from build123d import *

# Parameters (mm, degrees)
F0_R      = 5
F1_DEPTH  = 2
F2_R      = 4
F3_DEPTH  = 8
F4_R      = 6
F5_DEPTH  = 2
F7_DEPTH  = 2.5
F10_DEPTH = 8
F11_SIZE  = 1
F8_R      = 4
F8_R_2    = 3
F12_DEPTH = 3.1
F13_R     = 5
F13_R_2   = 4
F13_R_3   = 3
F14_DEPTH = 2
F16_DEPTH = 6
F17_SIZE  = 0.99999


# Not quite as in the source:
# - a fillet or chamfer is up to 0.001 mm smaller than in the source, because OpenCascade refuses the exact size


with BuildPart() as f1:
    # F0 (on Top) → F1 (new body)
    with BuildSketch(Plane.XY):
        Circle(F0_R)
    extrude(amount=F1_DEPTH)

    # F2 (on face) → F3 (join)
    with BuildSketch(Plane.XY.offset(2)):
        Circle(F2_R)
    extrude(amount=F3_DEPTH)

    # F4 (on face) → F5 (join)
    with BuildSketch(Plane.XY.offset(10)):
        Circle(F4_R)
    extrude(amount=F5_DEPTH)

    # F6 (on face) → F7 (join)
    with BuildSketch(Plane.XY.offset(12)):
        with BuildLine():
            ThreePointArc((6, 0), (5.9789831367, 0.5017575617), (5.9160797831, 1))
            Line((5.9160797831, 1), (4.5160797831, 1))
            Line((4.5160797831, 1), (4.5160797831, -1))
            Line((4.5160797831, -1), (5.9160797831, -1))
            ThreePointArc((5.9160797831, -1), (5.9789831367, -0.5017575617), (6, 0))
        make_face()
        with BuildLine():
            Line((-4.5160797831, 1), (-5.9160797831, 1))
            ThreePointArc((-5.9160797831, 1), (-6, 0), (-5.9160797831, -1))
            Line((-5.9160797831, -1), (-4.5160797831, -1))
            Line((-4.5160797831, -1), (-4.5160797831, 1))
        make_face()
    extrude(amount=F7_DEPTH)

    # F9 (on face) → F10 (cut)
    with BuildSketch(Plane(origin=(0, 0, 0), x_dir=(1, 0, 0), z_dir=(0, 0, -1))):
        with BuildLine():
            ThreePointArc((1.6, 2.6), (0, 3.0528675045), (-1.6, 2.6))
            Line((-1.6, 2.6), (-1.6, -2.6))
            ThreePointArc((-1.6, -2.6), (0, -3.0528675045), (1.6, -2.6))
            Line((1.6, -2.6), (1.6, 2.6))
        make_face()
    extrude(amount=-F10_DEPTH, mode=Mode.SUBTRACT)

    # F11
    f11_edges = [f1.edges().sort_by_distance(p)[0] for p in [
        (-5, 0, 0),
    ]]
    chamfer(f11_edges, length=F11_SIZE)

    # F8 (on face) → F12 (join)
    with BuildSketch(Plane.XY.offset(12)):
        Circle(F8_R)
        Circle(F8_R_2, mode=Mode.SUBTRACT)
    extrude(amount=F12_DEPTH)

    # F13 (on face) → F14 (join)
    with BuildSketch(Plane.XY.offset(15.1)):
        Circle(F13_R)
        Circle(F13_R_2, mode=Mode.SUBTRACT)
        Circle(F13_R_2)
        Circle(F13_R_3, mode=Mode.SUBTRACT)
    extrude(amount=F14_DEPTH)

    # F15 (on face) → F16 (cut)
    with BuildSketch(Plane.XY.offset(17.1)):
        with BuildLine():
            Line((-2.8284271247, 1), (-4.8989794856, 1))
            ThreePointArc((-4.8989794856, 1), (-5, 0), (-4.8989794856, -1))
            Line((-4.8989794856, -1), (-2.8284271247, -1))
            ThreePointArc((-2.8284271247, -1), (-3, 0), (-2.8284271247, 1))
        make_face()
        with BuildLine():
            ThreePointArc((0.9908586892, 4.9008365672), (-0.0278443772, 4.9999224685), (-1.0453806817, 4.8894968279))
            Line((-1.0453806817, 4.8894968279), (-1.0261823806, 2.819033473))
            ThreePointArc((-1.0261823806, 2.819033473), (-0.0085441177, 2.999987833), (1.0101083624, 2.8248329324))
            Line((1.0101083624, 2.8248329324), (0.9908586892, 4.9008365672))
        make_face()
        with BuildLine():
            ThreePointArc((5, 0), (4.974680765, 0.50254481), (4.8989794856, 1))
            Line((4.8989794856, 1), (2.8284271247, 1))
            ThreePointArc((2.8284271247, 1), (2.956795679, 0.5073059362), (3, 0))
            ThreePointArc((3, 0), (2.956795679, -0.5073059362), (2.8284271247, -1))
            Line((2.8284271247, -1), (4.8989794856, -1))
            ThreePointArc((4.8989794856, -1), (4.974680765, -0.50254481), (5, 0))
        make_face()
        with BuildLine():
            Line((-0.9737316464, -2.8375776079), (-0.9545333452, -4.9080409628))
            ThreePointArc((-0.9545333452, -4.9080409628), (0.0648756616, -4.9995790971), (1.0815661863, -4.8816200779))
            Line((1.0815661863, -4.8816200779), (1.0623165131, -2.8056164431))
            ThreePointArc((1.0623165131, -2.8056164431), (0.0470871391, -2.9996304441), (-0.9737316464, -2.8375776079))
        make_face()
    extrude(amount=-F16_DEPTH, mode=Mode.SUBTRACT)

    # F17 (size 1 in the source; OpenCascade refuses exactly that, so slightly less here)
    f17_edges = [f1.edges().sort_by_distance(p)[0] for p in [
        (3.564895, -3.505927, 15.1),
        (-3.551887, 3.519105, 15.1),
        (-3.519105, -3.551887, 15.1),
        (3.564895, -3.505927, 17.1),
        (-3.519105, -3.551887, 17.1),
        (-3.551887, 3.519105, 17.1),
        (3.532234, 3.53883, 17.1),
        (3.532234, 3.53883, 15.1),
    ]]
    chamfer(f17_edges, length=F17_SIZE)


solid = f1.part
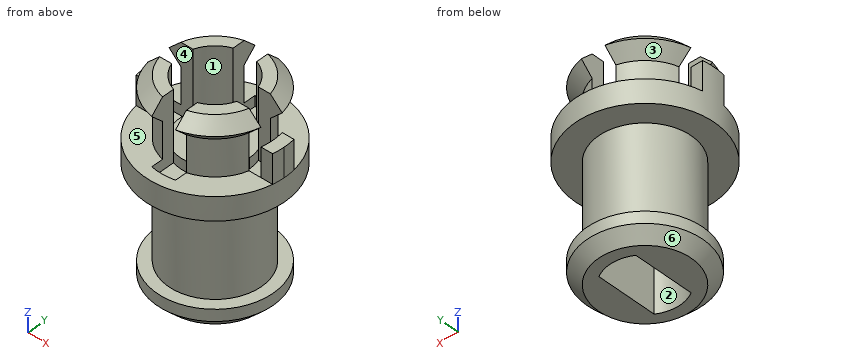
Can you work these out from the model? Positions are in its coordinate system, mm. Face numbers are marked on the shaded views. A direction names the side the tool comes from. Give positions to 0.01 mm unless a question says otherwise; leave off trailing zeros. Write each loop counter-clockwise with the first axis right and the second up, starting at its lowest first coordinate (ties: lowest second). Pieces come first, ordered by that corner, then holes. Notation, with made-up numbers: (-3, 57.5) -> (32, 57.5) arc R24 cw to (32, 70.5) -> close; hole circle Ø2 at (-4.75, 69). An arc over 180 degrees is marked (long way). Answer as a JSON object with one key per item and string values. Group by question number.
Item 1: We'd pull the mould along Z, two halves only. Please class the marked faces 4, 5 and 6: +Z half, -Z half, draft (parallel to the pull), parting line (faces both ways), or undercut.
Item 2: Please list where these lines run through material, in increasing order: line 1 (X direction, y = -4.25, z = 11.25); line 2 (Y direction, x = 2.5, z = 15.25); line 3 (Z direction, x = 5.25, y = -2.25). Write a range as [from, to].
Item 3: For the marked faces 1, 2 and 3, which set-ups out of +Z, -Z, +X, -X, +Y, -Y let a thin tool reach every point of the face, with its end or its side?
Item 4: Suppose I cut it at A-A (z = 2.25). Please give me the cut outline in (x, y).
Item 5: Suppose I cut it at C-C (z = 9.75). Please give me the cut outline in (x, y).
Item 6: Suppose I cut it at B-B (x = 0). Please give me the cut outline in (y, z), plus the area to 3 significant figures.
Item 7: I'm going to push flat-ended pins straight in: P1, Ø1.5, axis at x = 3.5, z = 2, coming from the +Y side; P2, Ø1.6, axis at x = 0.5, y = 0, coming from the -Z side; P3, Ø0.8, axis at x = 5.5, z = 13.5, coming from the -Y side. Where does each tip first touch, or does it pass through?
Findings:
{
 "1": {"face 4": "draft", "face 5": "undercut", "face 6": "-Z half"},
 "2": {"line 1": "x = [-4.24, -0.96], [1.08, 4.24]", "line 2": "y = [-3.31, -1.66], [1.66, 3.31]", "line 3": "z = [10, 12]"},
 "3": {"face 1": "+Z", "face 2": "-Z", "face 3": "-X, +Y"},
 "4": {"outline": "circle Ø8 at (0, 0); hole (-1.6, -2.6) arc R3.05 ccw to (1.6, -2.6) -> (1.6, 2.6) arc R3.05 ccw to (-1.6, 2.6) -> close"},
 "5": {"outline": "circle Ø8 at (0, 0)"},
 "6": {"outline": "(-6, 10) -> (-4, 10) -> (-4, 2) -> (-5, 2) -> (-5, 1) -> (-4, 0) -> (-3.05, 0) -> (-3.05, 8) -> (3.05, 8) -> (3.05, 0) -> (4, 0) -> (5, 1) -> (5, 2) -> (4, 2) -> (4, 10) -> (6, 10) -> (6, 12) -> (5, 12) -> (5, 11.1) -> (3, 11.1) -> (3, 12) -> (-3, 12) -> (-3, 11.1) -> (-5, 11.1) -> (-5, 12) -> (-6, 12) -> close", "area": "54.6 mm²"},
 "7": {"P1": "stops at y = 4.18", "P2": "stops at z = 8", "P3": "stops at y = -1"}
}
